Geometry: final body of the model. Coordinates: model frame, mm. A direction names the side the tool comes from. Coordinates: 2 decimals unless noted, no trailing zeros. Write each loop counter-clockwise with the first axis right and the second up, starting at its lowest first coordinate (ties: lowest second). Pieces come first, ordered by that corner, then holes. Notation, with made-up numbers: (74.5, 70.25) - (120.5, 70.25) arc R31 ccw to (120.5, 103.25) - close; hole circle Ø6 at (52, 33.5). An arc over 180 degrees is marked (long way). Put each result on its own line as item: value.
```python
from build123d import *

# Parameters (mm, degrees)
SKETCH1_W           = 101.6
SKETCH1_H           = 152.4
BOSS_EXTRUDE1_DEPTH = 6.35
SKETCH3_R           = 6.35
CUT_EXTRUDE2_DEPTH  = 3.175
SKETCH4_W           = 88.9
SKETCH4_H           = 139.7
CUT_EXTRUDE3_DEPTH  = 2.54
CUT_EXTRUDE4_REACH  = 185.272
SKETCH5_W           = 88.9
SKETCH5_H           = 1.27


with BuildPart() as part:
    # Sketch1 → Boss-Extrude1 (new body)
    with BuildSketch(Plane.XY):
        with Locations((50.8, 76.2)):
            Rectangle(SKETCH1_W, SKETCH1_H)
    extrude(amount=BOSS_EXTRUDE1_DEPTH)

    # Sketch3 → Cut-Extrude2 (cut)
    with BuildSketch(Plane.XY.offset(6.35)):
        with Locations((12.7, 139.7)):
            Circle(SKETCH3_R)
        with Locations((38.1, 139.7)):
            Circle(SKETCH3_R)
        with Locations((63.5, 139.7)):
            Circle(SKETCH3_R)
        with Locations((88.9, 139.7)):
            Circle(SKETCH3_R)
        with Locations(Location((88.9, 114.3, 0), (0, 0, 180))):
            Circle(SKETCH3_R)
        with Locations(Location((63.5, 114.3, 0), (0, 0, 180))):
            Circle(SKETCH3_R)
        with Locations(Location((38.1, 114.3, 0), (0, 0, 180))):
            Circle(SKETCH3_R)
        with Locations(Location((12.7, 114.3, 0), (0, 0, 180))):
            Circle(SKETCH3_R)
        with Locations((88.9, 88.9)):
            Circle(SKETCH3_R)
        with Locations((63.5, 88.9)):
            Circle(SKETCH3_R)
        with Locations((38.1, 88.9)):
            Circle(SKETCH3_R)
        with Locations((12.7, 88.9)):
            Circle(SKETCH3_R)
        with Locations(Location((88.9, 63.5, 0), (0, 0, 180))):
            Circle(SKETCH3_R)
        with Locations(Location((63.5, 63.5, 0), (0, 0, 180))):
            Circle(SKETCH3_R)
        with Locations(Location((38.1, 63.5, 0), (0, 0, 180))):
            Circle(SKETCH3_R)
        with Locations(Location((12.7, 63.5, 0), (0, 0, 180))):
            Circle(SKETCH3_R)
        with Locations((88.9, 38.1)):
            Circle(SKETCH3_R)
        with Locations((63.5, 38.1)):
            Circle(SKETCH3_R)
        with Locations((38.1, 38.1)):
            Circle(SKETCH3_R)
        with Locations((12.7, 38.1)):
            Circle(SKETCH3_R)
        with Locations(Location((88.9, 12.7, 0), (0, 0, 180))):
            Circle(SKETCH3_R)
        with Locations(Location((63.5, 12.7, 0), (0, 0, 180))):
            Circle(SKETCH3_R)
        with Locations(Location((38.1, 12.7, 0), (0, 0, 180))):
            Circle(SKETCH3_R)
        with Locations(Location((12.7, 12.7, 0), (0, 0, 180))):
            Circle(SKETCH3_R)
    extrude(amount=-CUT_EXTRUDE2_DEPTH, mode=Mode.SUBTRACT)

    # Sketch4 → Cut-Extrude3 (cut)
    with BuildSketch(Plane(origin=(0, 0, 0), x_dir=(-1, 0, 0), z_dir=(0, 0, -1))):
        with Locations((-50.8, 76.2)):
            Rectangle(SKETCH4_W, SKETCH4_H)
    extrude(amount=-CUT_EXTRUDE3_DEPTH, mode=Mode.SUBTRACT)

    # Sketch5 → Cut-Extrude4 (cut, up to next)
    with BuildSketch(Plane(origin=(0, 152.4, 0), x_dir=(1, 0, 0), z_dir=(0, 1, 0)), mode=Mode.PRIVATE) as cut_extrude4_sk1:
        with Locations((50.8, -1.905)):
            Rectangle(SKETCH5_W, SKETCH5_H)
    cut_extrude4_tool1 = extrude(cut_extrude4_sk1.sketch, amount=-CUT_EXTRUDE4_REACH, mode=Mode.PRIVATE) & part.part
    add(cut_extrude4_tool1.solids().sort_by_distance((50.8, 152.4, 1.905))[0], mode=Mode.SUBTRACT)


solid = part.part
```
1. Section query D-D (y = 53.5). Return loops of the section in (x, z), then the cut area to 3 significant figures.
Answer below:
outline: (0, 0) - (6.35, 0) - (6.35, 2.54) - (95.25, 2.54) - (95.25, 0) - (101.6, 0) - (101.6, 6.35) - (0, 6.35) - close
area: 419 mm²
2. Section query B-B (y = 12.7). Return loops of the section in (x, z) (3 decimals).
Answer below:
outline: (0, 0) - (6.35, 0) - (6.35, 2.54) - (95.25, 2.54) - (95.25, 0) - (101.6, 0) - (101.6, 6.35) - (95.25, 6.35) - (95.25, 3.175) - (82.55, 3.175) - (82.55, 6.35) - (69.85, 6.35) - (69.85, 3.175) - (57.15, 3.175) - (57.15, 6.35) - (44.45, 6.35) - (44.45, 3.175) - (31.75, 3.175) - (31.75, 6.35) - (19.05, 6.35) - (19.05, 3.175) - (6.35, 3.175) - (6.35, 6.35) - (0, 6.35) - close
3. Ray query, probe 1 along X at (y, z) = (89.5, 5.5); probe 2 along X at (y, z) = (132, 2.5); probe 3 along Y at (x, z) = (57.5, 0.75). Return the intervals inside material, ascending. Write a range as from..to.
Answer below:
probe 1: x = 0..6.38, 19.02..31.78, 44.42..57.18, 69.82..82.58, 95.22..101.6
probe 2: x = 0..6.35, 95.25..101.6
probe 3: y = 0..6.35, 146.05..152.4
4. Mould query, pull axis Y, two halves, no side actions, for faces 4 (the flat face through (50, 77, 6.35)), 5 (the flat face through (50, 152.4, 3)), 6 (the cylindrical face through (69.844, 12.421, 4.785)). Classes: +Y half, -Y half, draft (parallel to the pull), parting line (faces both ways), or undercut.
Answer below:
face 4: draft
face 5: +Y half
face 6: undercut
5. Pin query (flat end, axial travel): pin 1 Ø10 at (x, y) = (38.5, 13) entering from +Z (3 decimals); pin 2 Ø11.5 at (x, y) = (12.7, 139.7) entering from -Z. Return the tip coordinate at first contact, or that it passes through.
Answer below:
pin 1: stops at z = 3.175
pin 2: stops at z = 2.54
6. Section query C-C (x = 23.5). Return loops of the section in (y, z), then the cut area to 3 significant figures.
Answer below:
outline: (0, 0) - (6.35, 0) - (6.35, 2.54) - (152.4, 2.54) - (152.4, 6.35) - (0, 6.35) - close; (146.05, 0) - (152.4, 0) - (152.4, 1.27) - (146.05, 1.27) - close
area: 605 mm²
7. Set-up query: faces 1 (the flat face through (64, 114, 3.175)), 2 (the flat face through (5, 82, 0)), 3 (the flat face through (50, 149, 1.27)). Return all of +Z, -Z, +X, -X, +Y, -Y with unobstructed straight access to the full face (end or side cutting, diameter ignored); none if empty.
Answer below:
face 1: +Z
face 2: -Z, +X, -X, +Y, -Y
face 3: +Y
